Here's how the part is built. I have some questions about the finished solid (model axes, mm). A direction names the side the tool comes from. Round coordinates to 2 decimals unless told otherwise and drop trailing zeros. Write each loop counter-clockwise with the first axis right and the second up, starting at its lowest first coordinate (ties: lowest second). Pieces come first, ordered by that corner, then holes. Notation, with made-up numbers: M 78,30.25 L 97,30.25 A23 ccw 97,39.25 Z; hole C 57.25,-27.5 d4. An arc over 180 degrees is marked long. Write item = value, one per line. Start each with the question number.
(1) Will these pins go through, and if not, where does the flat tip stop? pin 1 Ø4.5 at (x, y) = (0, -50) entering from -Z (1 decimal); pin 2 Ø1 at (y, z) = (-12.5, 1.5) entering from +X; pin 3 Ø0.9 at (x, z) = (-11.5, 1) entering from +Y; pin 4 Ø0.9 at (x, z) = (-14, 1) entering from -Y.
(2) I want a section at A-A (x = 0). List the corners of the cut face in (y, z) for me, and give its area (3 significant figures).
(3) I want a section at B-B (z = 1.85). Give the number of separate pieces and of enclosed holes in the cut face, and give its area (3 significant figures).
(4) I want a section at C-C (x = -17.5). List the corners of the cut face in (y, z) for me.
(5) I need wall thicknesses on line 1 along X through (y, z) = (-4, 0.2); line 2 along X through (y, z) = (6.5, 0.2); line 3 along Y through (x, z) = (-34.5, 1.95). Which ranges of each line are inside material? Lowest first, please.
(6) If we mould it in two halves opening along X, with no side actions, what happens to faces 1 (the flat face through (11, 1, 3)), 2 (the cylindrical face through (-11.923, 53.692, 1.479)), 3 (the cylindrical face through (37.665, 36.313, 1.479))? For each: released by +X, released by -X, zero draft, split by the parting line, or undercut.
(7) On a 3-axis mill with a long thin cutter (end or side, diameter ignored), from which of +Z, -Z, +X, -X, +Y, -Y can I reach the whole of each face in a straight line? I mean faces 4 (the flat face through (11, 1, 0)), 5 (the flat face through (-27, 0, 2)). Say none if no direction works.
(8) I want a section at D-D (y = 5). List the corners of the cut face in (x, z) for me, and give its area (3 significant figures).
Autodesk Inventor part; units mm, degrees
ref_plane "YZ Plane" through (0, 0, 0) normal (1, 0, 0) x (0, 1, 0)
ref_plane "XZ Plane" through (0, 0, 0) normal (0, 1, 0) x (-1, 0, 0)
ref_plane "XY Plane" through (0, 0, 0) normal (0, 0, 1) x (1, 0, 0)
sketch "Boceto1" plane through (0, 0, 0) normal (0, 0, 1) x (1, 0, 0)
  circle A0 centre (0, 0) radius 55
  circle A1 centre (0, 0) radius 6.5
  circle A2 centre (0, 50) radius 2.5
  circle A3 centre (-35.3553, 35.3553) radius 2.5
  circle A4 centre (-50, 0) radius 2.5
  circle A5 centre (-35.3553, -35.3553) radius 2.5
  circle A6 centre (0, -50) radius 2.5
  circle A7 centre (35.3553, -35.3553) radius 2.5
  circle A8 centre (50, 0) radius 2.5
  circle A9 centre (35.3553, 35.3553) radius 2.5
  line L0 (0, 0) -> (14, 0)
  circle A10 centre (14, 5) radius 2.5
  circle A11 centre (14, -5) radius 2.5
  circle A12 centre (-34.5, 5) radius 2.5
  circle A13 centre (-34.5, -5) radius 2.5
  dimension "d7" = 360
extrude "Extrusión1" add sketch "Boceto1" along normal blind 3
sketch "Boceto2" plane through (0, 0, 3) normal (0, 0, 1) x (1, 0, 0)
  point P0 (0, 0)
sketch "Boceto3" plane through (0, 0, 3) normal (0, 0, 1) x (1, 0, 0)
  arc A0 (-4.4721, -9.5) -> (-4.4721, 9.5) centre (0, 0) ccw
  line L0 (-27, 0) -> (-27, -9.5)
  line L1 (-27, -9.5) -> (-27, 9.5)
  line L2 (-27, 9.5) -> (-4.4721, 9.5)
  line L3 (-27, -9.5) -> (-4.4721, -9.5)
extrude "Extrusión2" cut sketch "Boceto3" against normal blind 3
properties part number "Base1"
Returned:
q1.pin_1 = through
q1.pin_2 = 53.67
q1.pin_3 = 53.88
q1.pin_4 = -53.3
q2.outline = M -55,0 L -52.5,0 L -52.5,3 L -55,3 Z; M -47.5,0 L -10.5,0 L -10.5,3 L -47.5,3 Z; M 10.5,0 L 47.5,0 L 47.5,3 L 10.5,3 Z; M 52.5,0 L 55,0 L 55,3 L 52.5,3 Z
q2.area = 237 mm²
q3.separate_pieces = 1
q3.enclosed_holes = 13
q3.area = 8,580 mm²
q4.outline = M -52.14,0 L -9.5,0 L -9.5,3 L -52.14,3 Z; M 9.5,0 L 52.14,0 L 52.14,3 L 9.5,3 Z
q5.line_1 = -54.85 to -36.79, -32.21 to -27, 9.71 to 11.71, 16.29 to 54.85
q5.line_2 = -54.61 to -36.5, -32.5 to -27, 8.25 to 12, 16 to 54.61
q5.line_3 = -42.83 to -37.7, -33.01 to -7.5, -2.5 to 2.5, 7.5 to 33.01, 37.7 to 42.83
q6.face_1 = zero draft
q6.face_2 = split by the parting line
q6.face_3 = undercut
q7.face_4 = -Z, +X, -X, +Y, -Y
q7.face_5 = +Z, -Z
q8.outline = M -54.77,0 L -37,0 L -37,3 L -54.77,3 Z; M -32,0 L -27,0 L -27,3 L -32,3 Z; M 9.23,0 L 11.5,0 L 11.5,3 L 9.23,3 Z; M 16.5,0 L 54.77,0 L 54.77,3 L 16.5,3 Z
q8.area = 190 mm²
